from build123d import *

# Parameters (mm, degrees)
BOSS_EXTRUDE1_DEPTH = 5


with BuildPart() as part:
    # Sketch1 → Boss-Extrude1 (new body)
    with BuildSketch(Plane.XY):
        with BuildLine():
            ThreePointArc((9.444973397, -23.392615611), (0, -26.160254038), (-9.444973397, -23.392615611))
            Line((-9.444973397, -23.392615611), (-22.5, -12.086630926))
            Line((-22.5, -12.086630926), (-22.5, 34.44634768))
            Line((-22.5, 34.44634768), (-15.606601718, 41.339745962))
            Line((-15.606601718, 41.339745962), (15.606601718, 41.339745962))
            Line((15.606601718, 41.339745962), (22.5, 34.44634768))
            Line((22.5, 34.44634768), (22.5, -12.086630926))
            Line((22.5, -12.086630926), (9.444973397, -23.392615611))
        make_face()
        with BuildLine():
            Line((15, -8.660254038), (5, -17.320508076))
            ThreePointArc((5, -17.320508076), (0, -18.660254038), (-5, -17.320508076))
            Line((-5, -17.320508076), (-15, -8.660254038))
            Line((-15, -8.660254038), (-15, 31.339745962))
            Line((-15, 31.339745962), (-12.5, 33.839745962))
            Line((-12.5, 33.839745962), (12.5, 33.839745962))
            Line((12.5, 33.839745962), (15, 31.339745962))
            Line((15, 31.339745962), (15, -8.660254038))
        make_face(mode=Mode.SUBTRACT)
        Polygon((22.5, 174.44634768), (15.606601718, 167.552949398), (-15.606601718, 167.552949398), (-22.5, 174.44634768), (-22.5, 34.44634768), (-15.606601718, 41.339745962), (15.606601718, 41.339745962), (22.5, 34.44634768), align=None)
        with BuildLine():
            Line((22.5, 220.979326286), (9.444973397, 232.285310971))
            ThreePointArc((9.444973397, 232.285310971), (0, 235.052949398), (-9.444973397, 232.285310971))
            Line((-9.444973397, 232.285310971), (-22.5, 220.979326286))
            Line((-22.5, 220.979326286), (-22.5, 174.44634768))
            Line((-22.5, 174.44634768), (-15.606601718, 167.552949398))
            Line((-15.606601718, 167.552949398), (15.606601718, 167.552949398))
            Line((15.606601718, 167.552949398), (22.5, 174.44634768))
            Line((22.5, 174.44634768), (22.5, 220.979326286))
        make_face()
        with BuildLine():
            ThreePointArc((5, 226.213203436), (0, 227.552949398), (-5, 226.213203436))
            Line((-5, 226.213203436), (-15, 217.552949398))
            Line((-15, 217.552949398), (-15, 177.552949398))
            Line((-15, 177.552949398), (-12.5, 175.052949398))
            Line((-12.5, 175.052949398), (12.5, 175.052949398))
            Line((12.5, 175.052949398), (15, 177.552949398))
            Line((15, 177.552949398), (15, 217.552949398))
            Line((15, 217.552949398), (5, 226.213203436))
        make_face(mode=Mode.SUBTRACT)
        Polygon((-22.5, -12.086630926), (-22.5, 34.44634768), (-22.5, 46.339745962), (-27.5, 34.44634768), (-27.5, 29.44634768), (-27.5, -7.086630926), align=None)
        Polygon((22.5, -12.086630926), (27.5, -7.756503907), (27.5, 29.44634768), (22.5, 34.44634768), align=None)
        Polygon((22.5, 46.339745962), (22.5, 34.44634768), (27.5, 29.44634768), (27.5, 34.44634768), align=None)
        Polygon((22.5, 174.44634768), (22.5, 162.552949398), (27.5, 174.44634768), (27.5, 179.44634768), (27.5, 216.649199267), (22.5, 220.979326286), align=None)
        Polygon((-27.5, 174.44634768), (-22.5, 162.552949398), (-22.5, 174.44634768), (-22.5, 220.979326286), (-27.5, 215.979326286), (-27.5, 179.44634768), align=None)
    extrude(amount=BOSS_EXTRUDE1_DEPTH)


solid = part.part
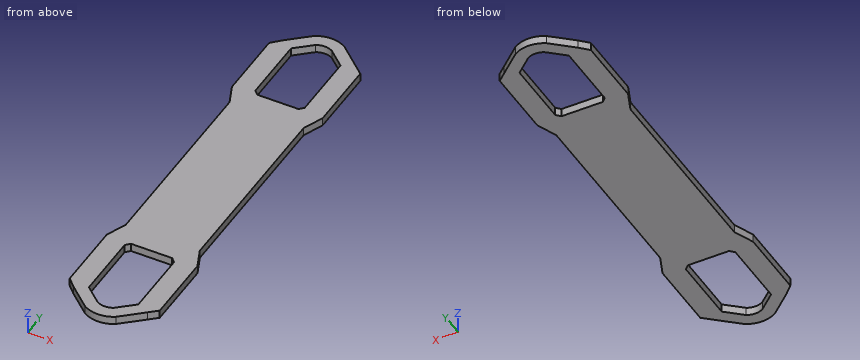
The listing builds one solid part. Answer for the finished solid, in the listing's coordinates (mm). Round coordinates to 2 decimals unless told otherwise and drop trailing zeros. Write each loop counter-clockwise with the first axis right and the second up, starting at its lowest first coordinate (ties: lowest second). Pieces come first, ordered by that corner, then holes. Notation, with made-up numbers: (-14.75, 5) - (32.25, 5) arc R35 ccw to (32.25, 41) - close; hole circle Ø10 at (20, 40.25). An arc over 180 degrees is marked (long way). Use a Markdown table: item, result. Add a question column.
1. Flat-ended cylindrical pins translate along their axes: P1, Ø2.5, axis at y = 103.5, z = 3.5, coming from the +X side; P2, Ø3, axis at x = -14.5, z = 3, coming from the -Y side; P3, Ø1, axis at y = 122, z = 1, coming from the -X side; P4, Ø12, axis at x = -21, y = 58.5, coming from the -Z side. Find the tip coordinate at first contact, or state that the pin passes through.
2. The part is cut by section D-D (y = 130). Write down the section's boundary in (x, z), and give its area (3 significant figures).
3. The part is cut by section A-A (y = 192.5). Write down the section's boundary in (x, z).
4. Consider line 1 (X direction, y = 187, z = 2.1); line 2 (Y direction, x = 11.5, z = 3.1); line 3 (X direction, y = 67.5, z = 4.6). Determine where each line is inside the solid, lowest interval first.
5. The part is cut by section C-C (z = 2). Give the number of separate pieces and of enclosed holes in the cut face, and give its area (3 significant figures).
6. The part is cut by section B-B (x = 2). Write down the section's boundary in (y, z).
Reported:
| question | item | result |
|---|---|---|
| 1 | P1 | x = 22.5 |
| 1 | P2 | y = -20.31 |
| 1 | P3 | x = -22.5 |
| 1 | P4 | z = 0 |
| 2 | outline | (-22.5, 0) - (22.5, 0) - (22.5, 5) - (-22.5, 5) - close |
| 2 | area | 225 mm^2 |
| 3 | outline | (-27.5, 0) - (-15, 0) - (-15, 5) - (-27.5, 5) - close; (15, 0) - (27.5, 0) - (27.5, 5) - (15, 5) - close |
| 4 | line 1 | -27.5 to -15, 15 to 27.5 |
| 4 | line 2 | -21.61 to -11.69, 33.84 to 175.05, 220.58 to 230.51 |
| 4 | line 3 | -22.5 to 22.5 |
| 5 | separate pieces | 1 |
| 5 | enclosed holes | 2 |
| 5 | area | 9,380 mm^2 |
| 6 | outline | (-26.05, 0) - (-18.46, 0) - (-18.46, 5) - (-26.05, 5) - close; (33.84, 0) - (175.05, 0) - (175.05, 5) - (33.84, 5) - close; (227.35, 0) - (234.94, 0) - (234.94, 5) - (227.35, 5) - close |
